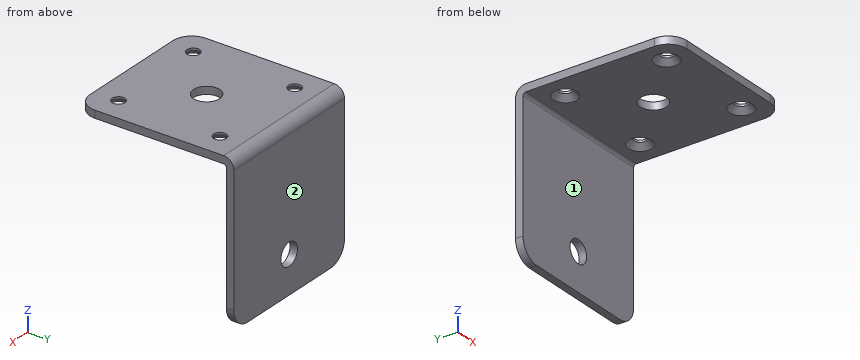
```python
from build123d import *

# Parameters (mm, degrees)
SKETCH_1_W                       = 40
SKETCH_1_H                       = 2
SM_BASE_FLANGE_1_DEPTH           = 40
CUT_EXTRUDE_1_REACH              = 58.604
SKETCH_3_R                       = 3
SM_EDGE_FLANGE_1_STRIP_W         = 9.4732
SM_EDGE_FLANGE_1_STRIP_H         = 2
SM_EDGE_FLANGE_1_STRIP_CUT_DEPTH = 40
SM_EDGE_FLANGE_1_DEPTH           = 40
FILLET_1_R                       = 5
HOLE_WIZARD_M3_1_AT_2_COUNT      = 2
HOLE_WIZARD_M3_1_AT_2_PITCH      = 27
HOLE_WIZARD_M3_1_AT_3_COUNT      = 2
HOLE_WIZARD_M3_1_AT_3_PITCH      = 38.183766184
HOLE_WIZARD_M3_1_AT_4_COUNT      = 2
HOLE_WIZARD_M3_1_AT_4_PITCH      = 27
HOLE_WIZARD_7_0_7_1_D            = 7
HOLE_WIZARD_7_0_7_1_DEPTH        = 2
HOLE_WIZARD_7_0_7_1_TIP          = 2.103012167


# Sheet-metal steps are written as plain solids
with BuildPart() as part:
    # Sketch 1 → 基材-凸緣1 (new body)
    with BuildSketch(Plane.XY):
        with Locations((20, -1)):
            Rectangle(SKETCH_1_W, SKETCH_1_H)
    extrude(amount=SM_BASE_FLANGE_1_DEPTH)

    # 草圖3 → 除料-伸長1 (cut, up to next)
    with BuildSketch(Plane(origin=(0, 0, 0), x_dir=(-1, 0, 0), z_dir=(0, 1, 0)), mode=Mode.PRIVATE) as cut_extrude_1_sk1:
        with Locations(Location((-20, 10, 0), (0, 0, 90))):
            Circle(SKETCH_3_R)
    cut_extrude_1_tool1 = extrude(cut_extrude_1_sk1.sketch, amount=-CUT_EXTRUDE_1_REACH, mode=Mode.PRIVATE) & part.part
    add(cut_extrude_1_tool1.solids().sort_by_distance((20, 0, 10))[0], mode=Mode.SUBTRACT)

    # 邊線-凸緣1 strip (across the edge) → 邊線-凸緣1 strip cut (cut)
    with BuildSketch(Plane(origin=(40, -2, 40), x_dir=(0, 0, -1), z_dir=(-1, 0, 0))):
        with Locations((-4, -1)):
            Rectangle(SM_EDGE_FLANGE_1_STRIP_W, SM_EDGE_FLANGE_1_STRIP_H)
    extrude(amount=SM_EDGE_FLANGE_1_STRIP_CUT_DEPTH, mode=Mode.SUBTRACT)

    # 邊線-凸緣1 section (across the edge) → 邊線-凸緣1 (add)
    with BuildSketch(Plane(origin=(40, -2, 40), x_dir=(0, 0, -1), z_dir=(-1, 0, 0))):
        with BuildLine():
            Line((-2, 0.7366), (-2, 40))
            Line((-2, 40), (0, 40))
            Line((0, 40), (0, 0.7366))
            ThreePointArc((0, 0.7366), (0.215745145, 0.215745145), (0.7366, 0))
            Line((0.7366, 0), (0.7366, -2))
            ThreePointArc((0.7366, -2), (-1.198468417, -1.198468417), (-2, 0.7366))
        make_face()
    extrude(amount=SM_EDGE_FLANGE_1_DEPTH)

    # 圓角1
    fillet_1_edges = [part.edges().sort_by_distance(p)[0] for p in [
        (0, -1, 0),
        (40, -42, 41),
        (0, -42, 41),
        (40, -1, 0),
    ]]
    fillet(fillet_1_edges, radius=FILLET_1_R)

    # 草圖7 → M3 平錐坑頭螺釘的錐孔1 (revolve, cut)
    with BuildSketch(Plane(origin=(33.5, -35.5, 40), x_dir=(0, 1, 0), z_dir=(1, 0, 0))):
        Polygon((0, 0), (0, 2), (1.7, 2), (1.7, 1.45), (3.15, 0), align=None)
    hole_wizard_m3_1 = revolve(axis=Axis((33.5, -35.5, 33.65), (0, 0, 1)), mode=Mode.SUBTRACT)

    # M3 平錐坑頭螺釘的錐孔1 at 2: M3 平錐坑頭螺釘的錐孔1 ×2
    with Locations(*[(0, i * HOLE_WIZARD_M3_1_AT_2_PITCH, 0) for i in range(1, HOLE_WIZARD_M3_1_AT_2_COUNT)]):
        add(hole_wizard_m3_1, mode=Mode.SUBTRACT)

    # M3 平錐坑頭螺釘的錐孔1 at 3: M3 平錐坑頭螺釘的錐孔1 ×2
    with Locations(*[Vector(-0.7071067811865475, 0.7071067811865477, -2.465626675858965e-15) * (i * HOLE_WIZARD_M3_1_AT_3_PITCH) for i in range(1, HOLE_WIZARD_M3_1_AT_3_COUNT)]):
        add(hole_wizard_m3_1, mode=Mode.SUBTRACT)

    # M3 平錐坑頭螺釘的錐孔1 at 4: M3 平錐坑頭螺釘的錐孔1 ×2
    with Locations(*[(-i * HOLE_WIZARD_M3_1_AT_4_PITCH, 0, 0) for i in range(1, HOLE_WIZARD_M3_1_AT_4_COUNT)]):
        add(hole_wizard_m3_1, mode=Mode.SUBTRACT)

    # Ø7.0 (7) 直徑孔1
    with Locations(Plane(origin=(0, 0, 40), x_dir=(-1, 0, 0), z_dir=(0, 0, -1))):
        with Locations((-20, -22)):
            Hole(HOLE_WIZARD_7_0_7_1_D / 2, depth=HOLE_WIZARD_7_0_7_1_DEPTH)
            with Locations((0, 0, -(HOLE_WIZARD_7_0_7_1_DEPTH + HOLE_WIZARD_7_0_7_1_TIP / 2))):  # 118° drill point
                Cone(0, HOLE_WIZARD_7_0_7_1_D / 2, HOLE_WIZARD_7_0_7_1_TIP, mode=Mode.SUBTRACT)


solid = part.part
```
Part model, mm, in its own coordinate system. Face numbers are marked on the shaded views. A direction names the side the tool comes from. Round coordinates to 2 decimals unless told otherwise and drop trailing zeros. Order: outer loops, then holes, each group sorted by start corner. A loop starts at its lowest first (then second) coordinate and runs counter-clockwise, first axis right, second up. Notation, with made-up numbers: M -6.5,-38.75 L 21.5,-38.75 A18 ccw 21.5,-15.75 Z; hole C 55,31 d8. An arc over 180 degrees is marked long. Answer in a Markdown table with one row per item. Add a question column.
Q1. 3-axis set-ups, long thin cutter, end or side, ignore diameter. For the marked faces 1 and 2: which of +Z, -Z, +X, -X, +Y, -Y reach the whole face in a straight line?
Q2. Wall check: L1, parallel to X at y = -35.5, z = 41.7; L2, parallel to Y at x = 33, z = 41; L3, parallel to Z at x = 21, y = -9. Give the ranges that are in metal, low to high. Write a range as from..to.
Q3. Cut at B-B on y = -8.5. Give the cut face in (x, z), and give its area (3 significant figures).
Q4. Cut at D-D on y = -22. Give the cut face in (x, z), and give its area (3 significant figures).
Q5. Cut at A-A on x = 20. Give the cut face in (y, z).
Q6. Cut at C-C on z = 10. Give the cut face in (x, y).
Q7. Pin check, flat tips, straight feed: pin 1 (2 mm diameter, centred on x = 7.5, z = 7.5, fed in from -Y); pin 2 (8 mm diameter, centred on x = 20, y = -22, fed in from -Z); pin 3 (2.5 mm diameter, centred on x = 33.5, y = -8.5, fed in from +Z); pin 4 (6 mm diameter, centred on x = 20.5, z = 10.5, fed in from +Y). Stop position of each tip, or through.
Established:
| question | item | result |
|---|---|---|
| 1 | face 1 | -Z, +X, -X, -Y |
| 1 | face 2 | +Z, -Z, +X, -X, +Y |
| 2 | L1 | x = 0..4.8, 8.2..31.8, 35.2..40 |
| 2 | L2 | y = -42..-37.59, -33.41..-10.59, -6.41..-0.62 |
| 2 | L3 | z = 40..42 |
| 3 | outline | M 0,40 L 3.35,40 L 4.8,41.45 L 4.8,42 L 0,42 Z; M 8.2,41.45 L 9.65,40 L 30.35,40 L 31.8,41.45 L 31.8,42 L 8.2,42 Z; M 35.2,41.45 L 36.65,40 L 40,40 L 40,42 L 35.2,42 Z |
| 3 | area | 62.2 mm2 |
| 4 | outline | M 0,40 L 16.5,40 L 16.5,42 L 0,42 Z; M 23.5,40 L 40,40 L 40,42 L 23.5,42 Z |
| 4 | area | 66.0 mm2 |
| 5 | outline | M -42,40 L -25.5,40 L -25.5,42 L -42,42 Z; M -18.5,40 L -2.74,40 A0.74 cw -2,39.26 L -2,13 L 0,13 L 0,39.26 A2.74 ccw -2.74,42 L -18.5,42 Z; M -2,0 L 0,0 L 0,7 L -2,7 Z |
| 6 | outline | M 0,-2 L 17,-2 L 17,0 L 0,0 Z; M 23,-2 L 40,-2 L 40,0 L 23,0 Z |
| 7 | pin 1 | stops at y = -2 |
| 7 | pin 2 | stops at z = 40 |
| 7 | pin 3 | passes through |
| 7 | pin 4 | stops at y = 0 |
